Answer from the drawing. Dimensions are ordinates in mm from the lowest x, y and z of the part. A direction names the side the tool comes from. Coordinates: 2 decimals unless noted, no trailing zeros. Loops run counter-clockwise (first coordinate to the right, second up) from the corner with the lowest first, then second, coordinate; pieces in that order, holes last. Notation, with made-up numbers: (42.5, -26.5) -> (71.5, -26.5) arc R20 ccw to (71.5, -1.5) -> close; hole circle Ø3 at (51, 57.25). An arc over 180 degrees is marked (long way). Answer as CSV lines item,"result".
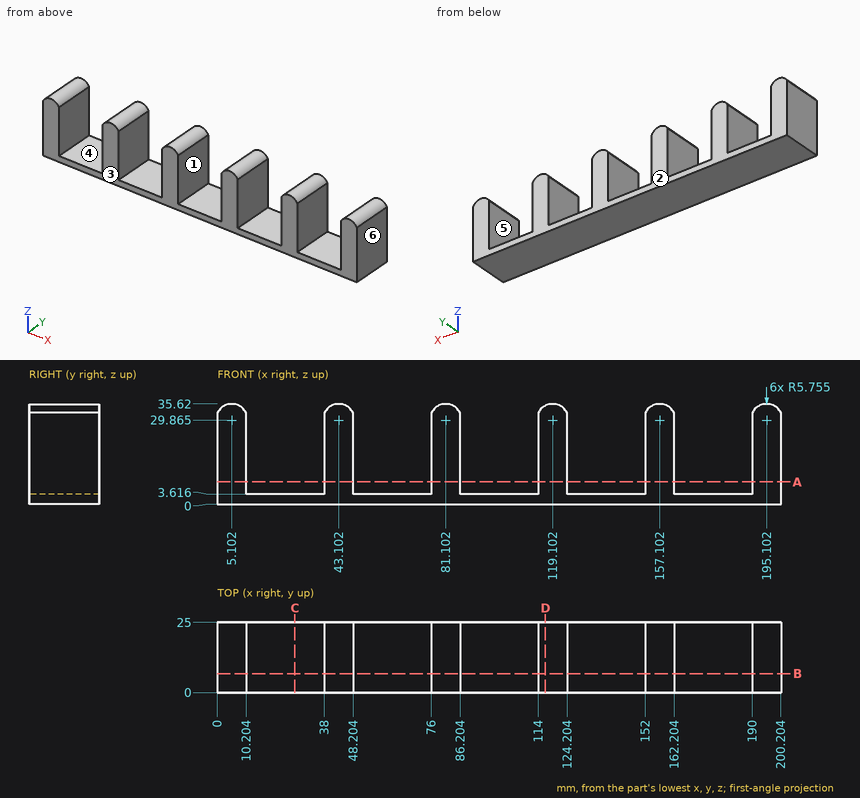
(1) A cutting plane is placed at C-C, the plane x = 27.5. Write down the section's boundary in (y, z) (1 decimal).
Computed values:
outline,"(0, 0) -> (25, 0) -> (25, 3.6) -> (0, 3.6) -> close"
(2) A cutting plane is placed at D-D, the plane x = 116.5. Write down the section's boundary in (y, z).
Computed values:
outline,"(0, 0) -> (25, 0) -> (25, 35) -> (0, 35) -> close"
(3) Flat-ended cylindrical pins translate along their axes: pin 1 Ø12.5 at (x, y) = (30.5, 14.5) entering from +Z; pin 2 Ø2 at (x, z) = (73, 5) entering from +Y. Find the tip coordinate at first contact, or state that the pin passes through.
Computed values:
pin 1,"z = 3.62"
pin 2,"through"
(4) A cutting plane is placed at A-A, the plane z = 8. Write down the section's boundary in (x, y) (1 decimal).
Computed values:
outline,"(0, 0) -> (10.2, 0) -> (10.2, 25) -> (0, 25) -> close; (38, 0) -> (48.2, 0) -> (48.2, 25) -> (38, 25) -> close; (76, 0) -> (86.2, 0) -> (86.2, 25) -> (76, 25) -> close; (114, 0) -> (124.2, 0) -> (124.2, 25) -> (114, 25) -> close; (152, 0) -> (162.2, 0) -> (162.2, 25) -> (152, 25) -> close; (190, 0) -> (200.2, 0) -> (200.2, 25) -> (190, 25) -> close"
(5) A cutting plane is placed at B-B, the plane y = 6.75. Write down the section's boundary in (x, z) (1 decimal).
Computed values:
outline,"(0, 0) -> (200.2, 0) -> (200.2, 32.5) arc R5.8 ccw to (190, 32.5) -> (190, 3.6) -> (162.2, 3.6) -> (162.2, 32.5) arc R5.8 ccw to (152, 32.5) -> (152, 3.6) -> (124.2, 3.6) -> (124.2, 32.5) arc R5.8 ccw to (114, 32.5) -> (114, 3.6) -> (86.2, 3.6) -> (86.2, 32.5) arc R5.8 ccw to (76, 32.5) -> (76, 3.6) -> (48.2, 3.6) -> (48.2, 32.5) arc R5.8 ccw to (38, 32.5) -> (38, 3.6) -> (10.2, 3.6) -> (10.2, 32.5) arc R5.8 ccw to (0, 32.5) -> close"
(6) Which of the six approach directions +Z, -Z, +X, -X, +Y, -Y give full straight-line access (tool end or side, diameter ignored) to the marked faces 1 and 2?
Computed values:
face 1,"+Z, +Y, -Y"
face 2,"+Z, -Z, +X, -X, +Y"
(7) For a pull along X with two mould halves and no side action, classify the marked faces 3, 4, 5 and 6 as pulls with the +X half, pulls with the -X half, needs draft (parallel to the pull), parting line crosses it, or undercut.
Computed values:
face 3,"needs draft"
face 4,"undercut"
face 5,"undercut"
face 6,"pulls with the +X half"
(8) Consider line 1 along X through (y, z) = (23, 28) (1 decimal); line 2 along X through (y, z) = (5, 33) (1 decimal); line 3 along Z through (x, y) = (137, 12.5) (1 decimal). Determine where each line is inside the solid, lowest interval first.
Computed values:
line 1,"0 to 10.2, 38 to 48.2, 76 to 86.2, 114 to 124.2, 152 to 162.2, 190 to 200.2"
line 2,"0.3 to 9.9, 38.3 to 47.9, 76.3 to 85.9, 114.3 to 123.9, 152.3 to 161.9, 190.3 to 199.9"
line 3,"0 to 3.6"
